The listing builds one solid part. Answer for the finished solid, in the listing's coordinates (mm). Coordinates: 2 decimals unless noted, no trailing zeros. Loops run counter-clockwise (first coordinate to the right, second up) from the corner with the lowest first, then second, coordinate; pieces in that order, holes last. Notation, with made-up numbers: M 6.25,-19.75 L 35.25,-19.75 A26 cw 35.25,9.25 Z; hole C 17.25,-31 d1. An arc over 180 degrees is marked long. Return JSON: item names as keys, results as strings. Group by question number.
1. Section A-A (y = -4.5) is taken. Write down the section's boundary in (x, z).
2. Section B-B (z = 0.5) is taken. Count the separate pieces of the cut face and the enclosed holes in it, then the cut area to 3 significant figures.
3. Given P1, Ø0.6, axis at y = -15.5, z = 1, coming from the +X side; P2, Ø18.5, axis at x = 51.64, y = -0.05, coming from the -Z side; P3, Ø1, axis at x = 86, z = 1, coming from the -Y side; P4, Ø1, axis at x = 13.5, z = 1, coming from the +Y side, each flat-ended and moving along its own axis, determine where each tip first touches the part or whether it passes through.
4. Straight lines are drawn through the part: L1, parallel to Y at x = 83.5, z = 0.65; L2, parallel to X at y = 20, z = 0.2; L3, parallel to X at y = 18.5, z = 0.5. For each, find the intervals that lie inside material, in ascending order. Write a range as from..to.
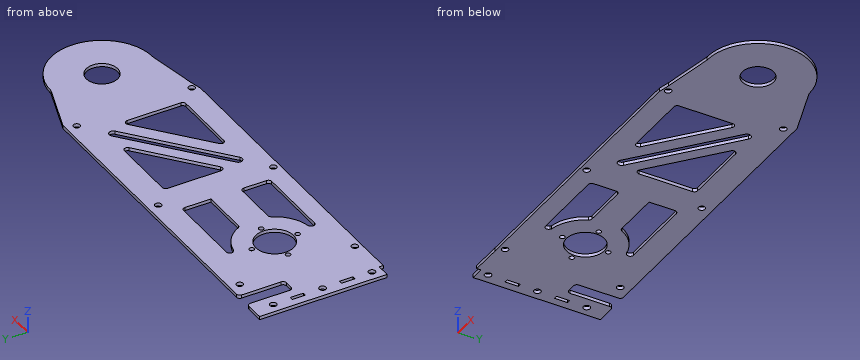
```python
from build123d import *

# Parameters (mm, degrees)
SKETCH_1_R          = 2.05
SKETCH_1_R_2        = 11.5
SKETCH_1_R_3        = 1.5
SKETCH_1_R_4        = 9.525
SKETCH_1_W          = 2.1
SKETCH_1_H          = 8.1
EXTRUDE_1_DEPTH     = 2
SKETCH_2_R          = 2
CUT_EXTRUDE_1_DEPTH = 4
FILLET_1_R          = 2


with BuildPart() as part:
    # 草图1 → 凸台-拉伸1 (new body)
    with BuildSketch(Plane.XY):
        with BuildLine():
            Line((-4.357142857, -0.045714286), (-4.357142857, 41.804285714))
            Line((-4.357142857, 41.804285714), (8.642857143, 41.804285714))
            Line((8.642857143, 41.804285714), (8.642857143, 13.804285714))
            Line((8.642857143, 13.804285714), (17.642857143, 13.804285714))
            Line((17.642857143, 13.804285714), (17.642857143, 41.804285714))
            Line((17.642857143, 41.804285714), (200.642857143, 41.804285714))
            Line((200.642857143, 41.804285714), (231.642857143, 30.954285714))
            ThreePointArc((231.642857143, 30.954285714), (262.642857143, -0.045714286), (231.642857143, -31.045714286))
            Line((231.642857143, -31.045714286), (200.656073527, -36.45591431))
            Line((200.656073527, -36.45591431), (193.846868021, -38.045714286))
            Line((193.846868021, -38.045714286), (22.465844759, -38.045714286))
            Line((22.465844759, -38.045714286), (3.792857143, -38.195714286))
            Line((3.792857143, -38.195714286), (3.792857143, -35.702553436))
            Line((3.792857143, -35.702553436), (-4.357142857, -35.702553436))
            Line((-4.357142857, -35.702553436), (-4.357142857, -0.045714286))
        make_face()
        with Locations((1.642857143, 29.954285714)):
            Circle(SKETCH_1_R, mode=Mode.SUBTRACT)
        with Locations((1.642857143, -0.045714286)):
            Circle(SKETCH_1_R, mode=Mode.SUBTRACT)
        with Locations((1.642857143, -30.045714286)):
            Circle(SKETCH_1_R, mode=Mode.SUBTRACT)
        with Locations((51.642857143, -0.045714286)):
            Circle(SKETCH_1_R_2, mode=Mode.SUBTRACT)
        with Locations((51.642857143, -14.045714286)):
            Circle(SKETCH_1_R_3, mode=Mode.SUBTRACT)
        with Locations((37.642857143, -0.045714286)):
            Circle(SKETCH_1_R_3, mode=Mode.SUBTRACT)
        with Locations((51.642857143, 13.954285714)):
            Circle(SKETCH_1_R_3, mode=Mode.SUBTRACT)
        with Locations((65.642857143, -0.045714286)):
            Circle(SKETCH_1_R_3, mode=Mode.SUBTRACT)
        with Locations((231.642857143, -0.045714286)):
            Circle(SKETCH_1_R_4, mode=Mode.SUBTRACT)
        with Locations((1.642857143, 14.954285714)):
            Rectangle(SKETCH_1_W, SKETCH_1_H, mode=Mode.SUBTRACT)
        with Locations((1.642857143, -15.045714286)):
            Rectangle(SKETCH_1_W, SKETCH_1_H, mode=Mode.SUBTRACT)
    extrude(amount=EXTRUDE_1_DEPTH)

    # 草图2 → 切除-拉伸1 (cut)
    with BuildSketch(Plane.XY.offset(2)):
        with Locations((26.642857143, 35.754285714)):
            Circle(SKETCH_2_R)
        with Locations((111.642857143, 35.754285714)):
            Circle(SKETCH_2_R)
        with Locations((196.642857143, 35.754285714)):
            Circle(SKETCH_2_R)
        with Locations((111.642857143, -34.245714286)):
            Circle(SKETCH_2_R)
        with Locations((196.642857143, -34.245714286)):
            Circle(SKETCH_2_R)
        with Locations((26.642857143, -34.245714286)):
            Circle(SKETCH_2_R)
        Polygon((187.542857143, -24.245714286), (140.41622539, -24.245714286), (187.542857143, 14.56445304), align=None)
        Polygon((122.542857143, 25.754285714), (169.669488896, 25.754285714), (122.542857143, -13.055881612), align=None)
        with BuildLine():
            Line((72.808867631, 8.954285714), (102.642857143, 8.954285714))
            Line((102.642857143, 8.954285714), (102.642857143, 26.754285714))
            Line((102.642857143, 26.754285714), (50.657939371, 26.754285714))
            Line((50.657939371, 26.754285714), (55.363054959, 22.651424922))
            ThreePointArc((55.363054959, 22.651424922), (65.846157695, 18.044787461), (72.808867631, 8.954285714))
        make_face()
        with BuildLine():
            Line((102.642857143, -9.045714286), (102.642857143, -26.845714286))
            Line((102.642857143, -26.845714286), (50.657939371, -26.845714286))
            Line((50.657939371, -26.845714286), (55.363054959, -22.742853493))
            ThreePointArc((55.363054959, -22.742853493), (65.846157695, -18.136216032), (72.808867631, -9.045714286))
            Line((72.808867631, -9.045714286), (102.642857143, -9.045714286))
        make_face()
        with BuildLine():
            Line((125.279005787, -19.870759717), (179.314122281, 24.628747983))
            ThreePointArc((179.314122281, 24.628747983), (182.731673921, 24.298017179), (182.400943117, 20.880465538))
            Line((182.400943117, 20.880465538), (128.365826624, -23.619042162))
            ThreePointArc((128.365826624, -23.619042162), (124.948274984, -23.288311358), (125.279005787, -19.870759717))
        make_face()
    extrude(amount=-CUT_EXTRUDE_1_DEPTH, mode=Mode.SUBTRACT)

    # 圆角1
    fillet_1_edges = [part.edges().sort_by_distance(p)[0] for p in [
        (72.808867631, 8.954285714, 1),
        (50.657939371, 26.754285714, 1),
        (102.642857143, 26.754285714, 1),
        (122.542857143, -13.055881612, 1),
        (122.542857143, 25.754285714, 1),
        (169.669488896, 25.754285714, 1),
        (187.542857143, 14.56445304, 1),
        (187.542857143, -24.245714286, 1),
        (140.41622539, -24.245714286, 1),
        (102.642857143, -26.845714286, 1),
        (50.657939371, -26.845714286, 1),
        (72.808867631, -9.045714286, 1),
        (102.642857143, -9.045714286, 1),
        (8.642857143, 41.804285714, 1),
        (8.642857143, 13.804285714, 1),
        (17.642857143, 13.804285714, 1),
        (17.642857143, 41.804285714, 1),
    ]]
    fillet(fillet_1_edges, radius=FILLET_1_R)


solid = part.part
```
Worked out:
{
 "1": {"outline": "M -4.36,0 L 41.04,0 L 41.04,2 L -4.36,2 Z; M 62.25,0 L 122.54,0 L 122.54,2 L 62.25,2 Z; M 132.93,0 L 143.94,0 L 143.94,2 L 132.93,2 Z; M 151.58,0 L 164.39,0 L 164.39,2 L 151.58,2 Z; M 187.54,0 L 223.22,0 L 223.22,2 L 187.54,2 Z; M 240.06,0 L 262.32,0 L 262.32,2 L 240.06,2 Z"},
 "2": {"separate pieces": "1", "enclosed holes": "22", "area": "15,400 mm^2"},
 "3": {"P1": "x = 258.69", "P2": "through", "P3": "y = -38.05", "P4": "y = 13.8"},
 "4": {"L1": "-38.05..-26.85, -9.05..8.95, 26.75..41.8", "L2": "-4.36..8.64, 17.64..62.92, 102.64..122.54, 162.68..173.69, 181.33..255.29", "L3": "-4.36..0.59, 2.69..8.64, 17.64..65.25, 102.64..122.54, 160.86..171.87, 179.51..256.48"}
}
